from build123d import *

# Parameters (mm, degrees)
BOX002_W     = 5
BOX002_H     = 5
BOX002_DEPTH = 10
BOX001_W     = 25
BOX001_H     = 25
BOX001_DEPTH = 5
BOX_W        = 15
BOX_H        = 15
BOX_DEPTH    = 10


with BuildPart() as cube002:
    # Box002 → Box002 (new body)
    with BuildSketch(Plane(origin=(25, 10, 0), x_dir=(1, 0, 0), z_dir=(0, 0, 1))):
        with Locations((2.5, 2.5)):
            Rectangle(BOX002_W, BOX002_H)
    extrude(amount=BOX002_DEPTH)


with BuildPart() as cut:
    # Box001 → Box001 (new body)
    with BuildSketch(Plane(origin=(15, 0, 0), x_dir=(1, 0, 0), z_dir=(0, 0, 1))):
        with Locations((12.5, 12.5)):
            Rectangle(BOX001_W, BOX001_H)
    extrude(amount=BOX001_DEPTH)

    # Cut: cut Cube002
    add(cube002.part, mode=Mode.SUBTRACT)


with BuildPart() as fusion:
    # Box → Box (new body)
    with BuildSketch(Plane(origin=(0, 5, 0), x_dir=(1, 0, 0), z_dir=(0, 0, 1))):
        with Locations((7.5, 7.5)):
            Rectangle(BOX_W, BOX_H)
    extrude(amount=BOX_DEPTH)

    # Fusion: union Cut
    add(cut.part)


solid = fusion.part
Read the model definition and answer for the solid it produces. Units are mm, in the model's axes. A direction names the side the tool comes from. Coordinates: 2 decimals unless noted, no trailing zeros. Loops run counter-clockwise (first coordinate to the right, second up) from the corner with the lowest first, then second, coordinate; pieces in that order, holes last. Notation, with made-up numbers: (16.25, 40.5) -> (21.25, 40.5) arc R12 cw to (21.25, 46.5) -> close; hole circle Ø4 at (9, -24.75). An arc over 180 degrees is marked (long way). Write item = value, one per line. Start each with the question number.
1) For faces 1 (the face through (15, 2, 2)), 2 (the face through (40, 12, 2)), 3 (the face through (27.3, 15.5, 5)), 4 (the face through (15, 22, 2)), 5 (the face through (30, 12, 2)), determine the directions among +Z, -Z, +X, -X, +Y, -Y from which every point of the face is accessible in a straight line to the end or side of a thin tool.
2) The part is cut by section D-D, the plane y = 17. Determine the outline of the cut face in (x, z), plus the area to 3 significant figures.
3) The part is cut by section B-B, the plane z = 3. Determine the outline of the cut face in (x, y), plus the area to 3 significant figures.
4) Given P1, Ø1, axis at y = 16, z = 8.5, coming from the +X side; P2, Ø3, axis at x = 5.5, z = 5.5, coming from the -Y side; P3, Ø2.5, axis at y = 3.5, z = 2, coming from the -X side, each flat-ended and moving along its own axis, determine where each tip first touches the part or whether it passes through.
5) The mould has two halves that part along Y. Classify faces 6 (the face through (7, 13, 10)), 7 (the face through (27, 15, 2)), 8 (the face through (27, 10, 2)), 9 (the face through (27, 25, 2)): pulls with the +Y half, pulls with the -Y half, needs draft (parallel to the pull), parting line crosses it, or undercut.
6) The part is cut by section C-C, the plane x = 29.5. Determine the outline of the cut face in (y, z).
7) Find the intervals of material crossed by L1, parallel to Z at x = 26, y = 1.75; L2, parallel to X at y = 14, z = 1.5; L3, parallel to Y at x = 11, z = 7.25, in increasing order. Write a range as from..to.
8) The part is cut by section A-A, the plane y = 11.25. Determine the outline of the cut face in (x, z).
Result:
q1.face_1 = +Z, -Z, -X, -Y
q1.face_2 = +Z, -Z, +X, +Y, -Y
q1.face_3 = +Z, +X, +Y, -Y
q1.face_4 = +Z, -Z, -X, +Y
q1.face_5 = +Z, -Z
q2.outline = (0, 0) -> (40, 0) -> (40, 5) -> (15, 5) -> (15, 10) -> (0, 10) -> close
q2.area = 275 mm²
q3.outline = (0, 5) -> (15, 5) -> (15, 0) -> (40, 0) -> (40, 25) -> (15, 25) -> (15, 20) -> (0, 20) -> close; hole (25, 10) -> (30, 10) -> (30, 15) -> (25, 15) -> close
q3.area = 825 mm²
q4.P1 = 15
q4.P2 = 5
q4.P3 = 15
q5.face_6 = needs draft
q5.face_7 = undercut
q5.face_8 = undercut
q5.face_9 = pulls with the +Y half
q6.outline = (0, 0) -> (10, 0) -> (10, 5) -> (0, 5) -> close; (15, 0) -> (25, 0) -> (25, 5) -> (15, 5) -> close
q7.L1 = 0..5
q7.L2 = 0..25, 30..40
q7.L3 = 5..20
q8.outline = (0, 0) -> (25, 0) -> (25, 5) -> (15, 5) -> (15, 10) -> (0, 10) -> close; (30, 0) -> (40, 0) -> (40, 5) -> (30, 5) -> close
